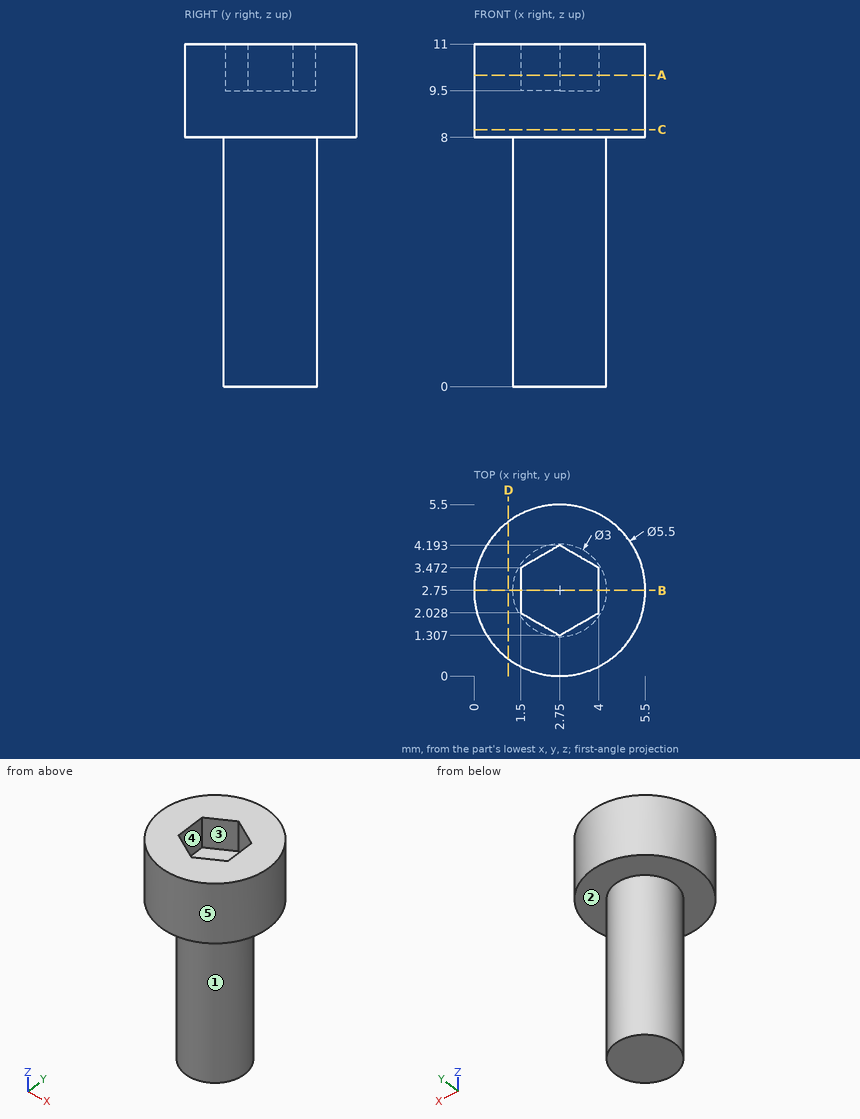
The figure shows three views and two pictorial views of one solid part (mm, origin at its lowest corner). Answer the questions. A direction names the side the tool comes from. Coordinates: 2 decimals unless noted, no trailing zeros. Write each loop counter-clockwise with the first axis right and the second up, starting at its lowest first coordinate (ties: lowest second). Pieces come first, ordered by that corner, then holes. Notation, with made-up numbers: M -14.5,84.5 L 13.5,84.5 A19 cw 13.5,121.5 Z; hole C 34,-19 d5. An arc over 180 degrees is marked long. Answer as CSV lines item,"result". Start each with the question number.
Item 1: Determine the mould class of the marked faces 1, 2 and 3 for opening direction X: released by +X, released by -X, zero draft, split by the parting line, or undercut.
Item 2: Consider L1, parallel to X at y = 2.8, z = 10; L2, parallel to Z at x = 0.65, y = 2.2; L3, parallel to Z at x = 1.65, y = 3.35. Determine where each line is inside the solid, lowest interval first.
Item 3: Section A-A on z = 10 is taken. Write down the section's boundary in (x, y).
Item 4: Section B-B on y = 2.75 is taken. Write down the section's boundary in (x, z).
Item 5: Section C-C on z = 8.25 is taken. Write down the section's boundary in (x, y).
Item 6: A flat-ended cylindrical pin translates along its axis: P1, Ø1.5, axis at x = 2.5, y = 3, coming from the +Z side. Find the tip coordinate at first contact, or state that the pin passes through.
Item 7: Section D-D on x = 1.1 is taken. Write down the section's boundary in (y, z), and give its area (3 significant figures).
Item 8: A tool of negligible diameter and unlimited length cuts with its end or side. For the marked faces 4 and 5, from which of +Z, -Z, +X, -X, +Y, -Y can it reach the whole face along a straight path? Write none if from no direction.
Checks:
1,face 1,"split by the parting line"
1,face 2,"zero draft"
1,face 3,"undercut"
2,L1,"x = 0 to 1.5, 4 to 5.5"
2,L2,"z = 8 to 11"
2,L3,"z = 0 to 9.5"
3,outline,"C 2.75,2.75 d5.5; hole M 1.5,2.03 L 2.75,1.31 L 4,2.03 L 4,3.47 L 2.75,4.19 L 1.5,3.47 Z"
4,outline,"M 0,8 L 1.25,8 L 1.25,0 L 4.25,0 L 4.25,8 L 5.5,8 L 5.5,11 L 4,11 L 4,9.5 L 1.5,9.5 L 1.5,11 L 0,11 Z"
5,outline,"C 2.75,2.75 d5.5"
6,P1,"stops at z = 9.5"
7,outline,"M 0.55,8 L 4.95,8 L 4.95,11 L 0.55,11 Z"
7,area,"13.2 mm²"
8,face 4,"+Z"
8,face 5,"+Z, -Z"
